Geometry: final body of the model. Coordinates: model frame, mm. Coordinates: 2 decimals unless noted, no trailing zeros. Order: outer loops, then holes, each group sorted by start corner. A loop starts at its lowest first (then second) coordinate and runs counter-clockwise, first axis right, second up. Notation, with made-up numbers: M -29.75,36.25 L 27.25,36.25 A8 ccw 27.25,50.25 Z; hole C 25.25,46 d9. An arc over 180 degrees is marked long. Use CSV: the item, a comma, the result in double quotes. Start each with the question number.
1. Section query C-C on x = -12.25. Return the cut outline in (y, z), and give its area (3 significant figures).
2. First-contact query: P1, Ø1.5, axis at x = -3, z = 15, coming from the +Y side. Flat tip, straight axial feed; report the tip coordinate or a pass-through.
3. Section query A-A on y = 0.1. Return the cut outline in (x, z).
4. Material intervals for line 1 (Z direction, x = -5.25, y = 0.15); line 2 (X direction, y = 0.35, z = 17); line 3 (Z direction, x = 12, y = 0.2), sorted ascending.
5. Section query B-B on z = 18.5. Return the cut outline in (x, y).
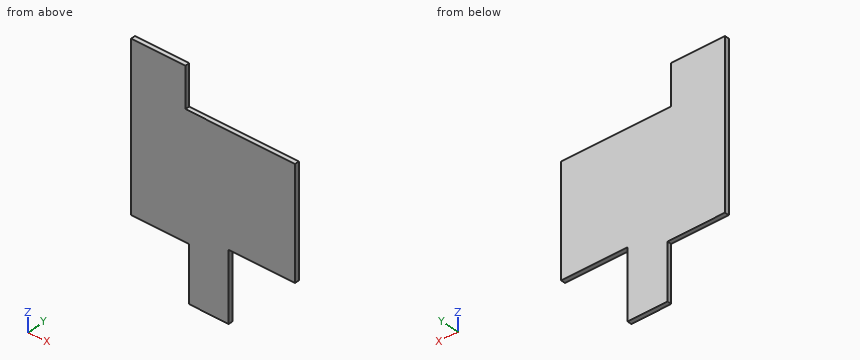
from build123d import *

# Parameters (mm, degrees)
BOSS_EXTRU_1_DEPTH = 0.4


with BuildPart() as part:
    # Esquisse1 → Boss.-Extru.1 (new body, symmetric)
    with BuildSketch(Plane(origin=(0, 0, 0), x_dir=(1, 0, 0), z_dir=(0, 1, 0))):
        Polygon((-15, -20), (-5.070958152, -20), (-5.070958152, -12.669744809), (15, -12.669744809), (15, 7.44690143), (2.85169362, 7.44690143), (2.85169362, 20), (-4.450924535, 20), (-4.450924535, 9.858143274), (-15, 9.858143274), align=None)
    extrude(amount=BOSS_EXTRU_1_DEPTH, both=True)


solid = part.part
Results list:
1,outline,"M -0.4,-9.86 L 0.4,-9.86 L 0.4,20 L -0.4,20 Z"
1,area,"23.9 mm²"
2,P1,"passes through"
3,outline,"M -15,-9.86 L -4.45,-9.86 L -4.45,-20 L 2.85,-20 L 2.85,-7.45 L 15,-7.45 L 15,12.67 L -5.07,12.67 L -5.07,20 L -15,20 Z"
4,line 1,"z = -9.86 to 20"
4,line 2,"x = -15 to -5.07"
4,line 3,"z = -7.45 to 12.67"
5,outline,"M -15,-0.4 L -5.07,-0.4 L -5.07,0.4 L -15,0.4 Z"
